```python
from build123d import *

# Parameters (mm, degrees)
SKETCH1_R           = 0.75
SKETCH1_R_2         = 1.5
BOSS_EXTRUDE1_DEPTH = 3
SKETCH2_R           = 3.5
CUT_EXTRUDE1_DEPTH  = 1.5
SKETCH3_R           = 4
BOSS_EXTRUDE2_DEPTH = 2.99
SKETCH4_R           = 2.5
CUT_EXTRUDE2_DEPTH  = 4
SKETCH5_R           = 5.5
SKETCH5_R_2         = 4
BOSS_EXTRUDE3_DEPTH = 3
CHAMFER1_SIZE       = 0.25


with BuildPart() as part:
    # Sketch1 → Boss-Extrude1 (new body)
    with BuildSketch(Plane(origin=(0, 0, 0), x_dir=(1, 0, 0), z_dir=(0, 1, 0))):
        with BuildLine():
            Line((-16, 6), (16, 6))
            ThreePointArc((16, 6), (22, 0), (16, -6))
            Line((16, -6), (-16, -6))
            ThreePointArc((-16, -6), (-22, 0), (-16, 6))
        make_face()
        with Locations((10, 0)):
            Circle(SKETCH1_R, mode=Mode.SUBTRACT)
        with Locations((13, 0)):
            Circle(SKETCH1_R, mode=Mode.SUBTRACT)
        with Locations((16, 0)):
            Circle(SKETCH1_R, mode=Mode.SUBTRACT)
        with Locations((19, 0)):
            Circle(SKETCH1_R, mode=Mode.SUBTRACT)
        with Locations((-19, 0)):
            Circle(SKETCH1_R, mode=Mode.SUBTRACT)
        with Locations((-16, 0)):
            Circle(SKETCH1_R, mode=Mode.SUBTRACT)
        with Locations((-13, 0)):
            Circle(SKETCH1_R, mode=Mode.SUBTRACT)
        with Locations((-10, 0)):
            Circle(SKETCH1_R, mode=Mode.SUBTRACT)
        Circle(SKETCH1_R_2, mode=Mode.SUBTRACT)
    extrude(amount=BOSS_EXTRUDE1_DEPTH)

    # Sketch2 → Cut-Extrude1 (cut)
    with BuildSketch(Plane(origin=(0, 0, 0), x_dir=(-1, 0, 0), z_dir=(0, -1, 0))):
        Circle(SKETCH2_R)
    extrude(amount=-CUT_EXTRUDE1_DEPTH, mode=Mode.SUBTRACT)

    # Sketch3 → Boss-Extrude2 (add)
    with BuildSketch(Plane(origin=(0, 3, 0), x_dir=(1, 0, 0), z_dir=(0, 1, 0))):
        Circle(SKETCH3_R)
    extrude(amount=BOSS_EXTRUDE2_DEPTH)

    # Sketch4 → Cut-Extrude2 (cut)
    with BuildSketch(Plane(origin=(0, 5.99, 0), x_dir=(1, 0, 0), z_dir=(0, 1, 0))):
        Circle(SKETCH4_R)
    extrude(amount=-CUT_EXTRUDE2_DEPTH, mode=Mode.SUBTRACT)

    # Sketch5 → Boss-Extrude3 (add)
    with BuildSketch(Plane(origin=(0, 3, 0), x_dir=(1, 0, 0), z_dir=(0, 1, 0))):
        Circle(SKETCH5_R)
        Circle(SKETCH5_R_2, mode=Mode.SUBTRACT)
    extrude(amount=BOSS_EXTRUDE3_DEPTH)

    # Chamfer1
    chamfer1_edges = [part.edges().sort_by_distance(p)[0] for p in [
        (-5.5, 6, 0),
    ]]
    chamfer(chamfer1_edges, length=CHAMFER1_SIZE)


solid = part.part
```
Input: part model. Units: mm. Frame: model coordinates. A direction names the side the tool comes from. Give positions to 0.01 mm unless a question says otherwise; leave off trailing zeros. Order: outer loops, then holes, each group sorted by start corner. A loop starts at its lowest first (then second) coordinate and runs counter-clockwise, first axis right, second up. Notation, with made-up numbers: M 2,-31.75 L 24,-31.75 A12 ccw 24,-9.75 Z; hole C 55,-30 d2. An arc over 180 degrees is marked long. One line per question, with ' | ' between items. Start each with the question number.
1. Section query C-C (x = -19). Return the cut outline in (y, z).
2. Section query A-A (x = -13). Return the cut outline in (y, z), and give its area (3 significant figures).
3. First-contact query: pin 1 Ø1.2 at (x, z) = (19, 0) entering from +Y; pin 2 Ø2 at (x, z) = (-19, 0) entering from +Y; pin 3 Ø6 at (x, z) = (0, 0) entering from +Y; pin 4 Ø2 at (y, z) = (2, 2.5) entering from -X. Flat tips, straight axial feed; report the tip coordinate or a pass-through.
4. Pull-direction query (Z, two-part tool) for faces 1 (the face through (0, 0, -4)), 2 (the face through (-16.595, 1.479, 0.456)), 3 (the face through (22, 1, 0)); classes: released by +Z, released by -Z, zero draft, split by the parting line, or undercut.
5. Material intervals for probe 1 along Y at (x, z) = (-13, -1.25); probe 2 along Z at (x, y) = (-3, 0.5); probe 3 along Z at (x, y) = (-19, 0.65), sorted ascending. Write a range as [from, to].
6. Access query for faces 4 (the face through (-13.75, 1.48, -0.03)), 5 (the face through (-3.233, 0.74, 1.341)), 6 (the face through (0, 1.99, 2)). Directions: +Z, -Z, +X, -X, +Y, -Y. A direction counts if a zero-diameter tool reaches every point of the face in a straight line with its end or side. Return the directions, or none.
Here are the results:
1) outline: M 0,-5.2 L 3,-5.2 L 3,-0.75 L 0,-0.75 Z; M 0,0.75 L 3,0.75 L 3,5.2 L 0,5.2 Z
2) outline: M 0,-6 L 3,-6 L 3,-0.75 L 0,-0.75 Z; M 0,0.75 L 3,0.75 L 3,6 L 0,6 Z | area: 31.5 mm²
3) pin 1: through | pin 2: y = 3 | pin 3: y = 5.99 | pin 4: x = -21.81
4) face 1: zero draft | face 2: undercut | face 3: split by the parting line
5) probe 1: [0, 3] | probe 2: [-6, -1.8], [1.8, 6] | probe 3: [-5.2, -0.75], [0.75, 5.2]
6) face 4: +Y, -Y | face 5: -Y | face 6: +Y
